```python
from build123d import *

# Parameters (mm, degrees)
F2_W     = 8.328109514
F2_H     = 5.4839188233
F3_DEPTH = 40.001
F4_SIZE  = 1
F5_F1_R  = 1
F5_F2_R  = 1
F5_F3_R  = 1


with BuildPart() as f1:
    # F0 (on Front) → F1 (revolve)
    with BuildSketch(Plane.XZ):
        with BuildLine():
            Line((0, 15), (0, 0))
            Line((0, 0), (40, 0))
            Line((40, 0), (40, 15))
            ThreePointArc((40, 15), (38.8284271247, 17.8284271247), (36, 19))
            Line((36, 19), (29, 19))
            ThreePointArc((29, 19), (26.1715728753, 17.8284271247), (25, 15))
            Line((25, 15), (25, 10))
            Line((25, 10), (0, 15))
        make_face()
    revolve(axis=Axis((20, 0, 0), (-1, 0, 0)))

    # F2 (on face) → F3 (cut, through all)
    with BuildSketch(Plane(origin=(0, 0, 0), x_dir=(0, -1, 0), z_dir=(-1, 0, 0))):
        Rectangle(F2_W, F2_H)
    extrude(amount=-F3_DEPTH, mode=Mode.SUBTRACT)

    # F4
    f4_edges = [f1.edges().sort_by_distance(p)[0] for p in [
        (0, 0, -15),
    ]]
    chamfer(f4_edges, length=F4_SIZE)

    # F5: fillet of radius 1 on 8 edges, made by hand

    # F5_f1
    f5_f1_edges = [f1.edges().sort_by_distance(p)[0] for p in [
        (20, -4.164054757, 2.7419594117),
        (20, -4.164054757, -2.7419594117),
        (20, 4.164054757, 2.7419594117),
        (20, 4.164054757, -2.7419594117),
    ]]
    fillet(f5_f1_edges, radius=F5_F1_R)

    # F5_f2
    f5_f2_edges = [f1.edges().sort_by_distance(p)[0] for p in [
        (0, -4.164054757, 0),
        (0, 4.164054757, 0),
        (0, 3.8711615382, 2.4490661928),
        (0, 3.8711615382, -2.4490661928),
        (0, -3.8711615382, -2.4490661928),
        (0, -3.8711615382, 2.4490661928),
    ]]
    fillet(f5_f2_edges, radius=F5_F2_R)

    # F5_f3
    f5_f3_edges = [f1.edges().sort_by_distance(p)[0] for p in [
        (40, -4.164054757, 0),
        (40, 0, -2.7419594117),
        (40, -3.8711615382, -2.4490661928),
        (40, 3.8711615382, -2.4490661928),
        (40, -3.8711615382, 2.4490661928),
    ]]
    fillet(f5_f3_edges, radius=F5_F3_R)


solid = f1.part
```
Build history of the part. All positions in model axes, mm. A direction names the side the tool comes from. Coordinates: 2 decimals unless noted, no trailing zeros. Order: outer loops, then holes, each group sorted by start corner. A loop starts at its lowest first (then second) coordinate and runs counter-clockwise, first axis right, second up. Notation, with made-up numbers: (64.5, 79) -> (112.5, 79) arc R5 ccw to (112.5, 84) -> close; hole circle Ø7 at (31.5, 23). An arc over 180 degrees is marked (long way). Answer in a Markdown table with one row per item. Add a question column.
Q1. Wall check: line 1 along Y through (x, z) = (37, -1); line 2 along Z through (x, y) = (27, -1.5); line 3 along Y through (x, z) = (25.5, -6). Give the ranges that are in metal, low to high. Write a range as [from, to].
Q2. Band-saw the part on A-A, the plane y = 0. List the corners of the cut face in (x, z), then the cut area to 3 significant figures.
Q3. Band-saw the part on C-C, the plane x = 7. List the corners of the cut face in (y, z), then the cut area to 3 significant figures.
Q4. Mould opens along Y. For faces 4 (the face through (0, -6, 0)), 5 (the face through (15.491, 3.575, 11.352)), 6 (the face through (20, 0, 2.742)) say: +Y half, -Y half, draft (parallel to the pull), parting line (faces both ways), or undercut.
Q5. Band-saw the part on B-B, the plane z = 0. List the corners of the cut face in (x, y).
Q6. Band-saw the part on D-D, the plane x = 37. List the corners of the cut face in (y, z), then the cut area to 3 significant figures.
Q7. Drop flat-ended pins along their axis: pin 1 (3 mm diameter, centred on x = 8, y = 10.5, fed in from +Z); pin 2 (3 mm diameter, centred on x = 26, y = 0, fed in from -Z); pin 3 (3 mm diameter, centred on x = 18, z = -0.5, fed in from -Y). Give the stop position or say it passes through.
Q8. Which spindle directions (+Z, -Z, +X, -X, +Y, -Y) get a long thin tool onto all of the face, cutting with end or side? Do faces 1 (the face through (25, -10, 3)), 2 (the face through (20, 0, -2.742)), 3 (the face through (40, -6, 0)). Say none if no direction does.
Answers follow:
| question | item | result |
|---|---|---|
| 1 | line 1 | [-18.85, -4.16], [4.16, 18.85] |
| 1 | line 2 | [-18.4, -2.74], [2.74, 18.4] |
| 1 | line 3 | [-15.84, 15.84] |
| 2 | outline | (0, -14) -> (0.98, -14.8) -> (25, -10) -> (25, -15) arc R4 ccw to (29, -19) -> (36, -19) arc R4 ccw to (40, -15) -> (40, -3.74) arc R1 ccw to (39, -2.74) -> (1, -2.74) arc R1 ccw to (0, -3.74) -> close; (0, 3.74) arc R1 ccw to (1, 2.74) -> (39, 2.74) arc R1 ccw to (40, 3.74) -> (40, 15) arc R4 ccw to (36, 19) -> (29, 19) arc R4 ccw to (25, 15) -> (25, 10) -> (0.98, 14.8) -> (0, 14) -> close |
| 2 | area | 960 mm^2 |
| 3 | outline | circle Ø27.2 at (0, 0); hole (-4.16, -1.74) arc R1 ccw to (-3.16, -2.74) -> (3.16, -2.74) arc R1 ccw to (4.16, -1.74) -> (4.16, 1.74) arc R1 ccw to (3.16, 2.74) -> (-3.16, 2.74) arc R1 ccw to (-4.16, 1.74) -> close |
| 3 | area | 536 mm^2 |
| 4 | face 4 | draft |
| 4 | face 5 | parting line |
| 4 | face 6 | undercut |
| 5 | outline | (0, -14) -> (0.98, -14.8) -> (25, -10) -> (25, -15) arc R4 ccw to (29, -19) -> (36, -19) arc R4 ccw to (40, -15) -> (40, -5.16) arc R1 ccw to (39, -4.16) -> (1, -4.16) arc R1 ccw to (0, -5.16) -> close; (0, 5.16) arc R1 ccw to (1, 4.16) -> (39, 4.16) arc R1 ccw to (40, 5.16) -> (40, 15) arc R4 ccw to (36, 19) -> (29, 19) arc R4 ccw to (25, 15) -> (25, 10) -> (0.98, 14.8) -> (0, 14) -> close |
| 6 | outline | circle Ø37.75 at (0, 0); hole (-4.16, -1.74) arc R1 ccw to (-3.16, -2.74) -> (3.16, -2.74) arc R1 ccw to (4.16, -1.74) -> (4.16, 1.74) arc R1 ccw to (3.16, 2.74) -> (-3.16, 2.74) arc R1 ccw to (-4.16, 1.74) -> close |
| 6 | area | 1,070 mm^2 |
| 7 | pin 1 | z = 9.99 |
| 7 | pin 2 | z = -18.71 |
| 7 | pin 3 | y = -11.69 |
| 8 | face 1 | none |
| 8 | face 2 | +X, -X |
| 8 | face 3 | +Z, -Z, +X, +Y, -Y |
